Geometry check sheet. Reference: the model listing, model coordinates, mm. Face numbers are marked on the shaded views. A direction names the side the tool comes from. Round coordinates to 2 decimals unless told otherwise and drop trailing zeros. Write each loop counter-clockwise with the first axis right and the second up, starting at its lowest first coordinate (ties: lowest second). Pieces come first, ordered by that corner, then holes. Notation, with made-up numbers: (64, -2) -> (120, -2) arc R19 ccw to (120, 33) -> close; hole circle Ø1 at (-35.5, 8.5). An arc over 180 degrees is marked (long way). One line per question, with ' | ' between items.
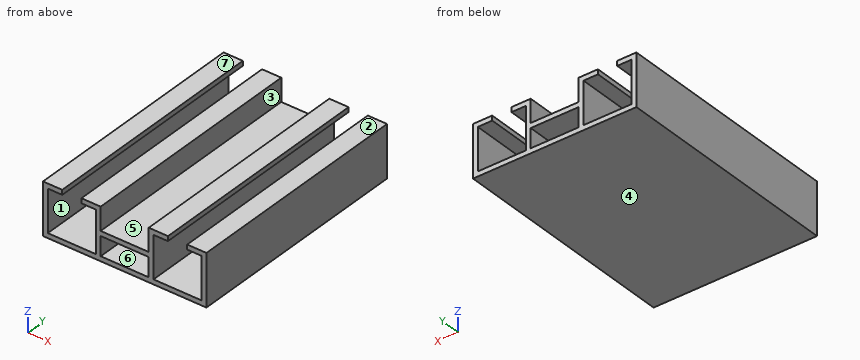
```python
from build123d import *

# Parameters (mm, degrees)
F0_W     = 25
F0_H     = 10
F1_DEPTH = 60


with BuildPart() as f1:
    # F0 (on Front) → F1 (new body, symmetric)
    with BuildSketch(Plane.XZ):
        Polygon((42.5, -17.5), (42.5, 9.5), (32.5, 9.5), (32.5, 7), (40, 7), (40, -15), (15, -15), (15, 7), (22.5, 7), (22.5, 9.5), (12.5, 9.5), (12.5, -2.5), (-12.5, -2.5), (-12.5, 9.5), (-22.5, 9.5), (-22.5, 7), (-15, 7), (-15, -15), (-40, -15), (-40, 7), (-32.5, 7), (-32.5, 9.5), (-42.5, 9.5), (-42.5, -17.5), align=None)
        with Locations((0, -10)):
            Rectangle(F0_W, F0_H, mode=Mode.SUBTRACT)
    extrude(amount=F1_DEPTH, both=True)


solid = f1.part
```
(1) Sectioned sample at A-A on z = -7.75. Record the cut outline in (x, y), then the cut area to 3 significant figures.
Resolved:
outline: (-42.5, -60) -> (-40, -60) -> (-40, 60) -> (-42.5, 60) -> close; (-15, -60) -> (-12.5, -60) -> (-12.5, 60) -> (-15, 60) -> close; (12.5, -60) -> (15, -60) -> (15, 60) -> (12.5, 60) -> close; (40, -60) -> (42.5, -60) -> (42.5, 60) -> (40, 60) -> close | area: 1,200 mm2
(2) Material ranges on line 1 (X direction, y = 48, z = 8.75); line 2 (X direction, y = 38.5, z = -11.25); line 3 (X direction, y = 17, z = -4.5), recorded low to high.
Resolved:
line 1: x = -42.5 to -32.5, -22.5 to -12.5, 12.5 to 22.5, 32.5 to 42.5 | line 2: x = -42.5 to -40, -15 to -12.5, 12.5 to 15, 40 to 42.5 | line 3: x = -42.5 to -40, -15 to 15, 40 to 42.5
(3) Access from +Z, -Z, +X, -X, +Y, -Y to the whole of each face (thin tool, end or side, straight path). Record for the marked faces 5, 6 and 7.
Resolved:
face 5: +Z, +Y, -Y | face 6: +Y, -Y | face 7: +Z, +X, -X, +Y, -Y
(4) Draft check along Z on the marked faces 1, 2, 3 and 4. Enter one of: +Z half, -Z half, draft (parallel to the pull), parting line (faces both ways), or undercut.
Resolved:
face 1: undercut | face 2: +Z half | face 3: draft | face 4: -Z half
(5) Sectioned sample at C-C on y = -7.5. Record the cut outline in (x, z), then the cut area to 3 significant figures.
Resolved:
outline: (-42.5, -17.5) -> (42.5, -17.5) -> (42.5, 9.5) -> (32.5, 9.5) -> (32.5, 7) -> (40, 7) -> (40, -15) -> (15, -15) -> (15, 7) -> (22.5, 7) -> (22.5, 9.5) -> (12.5, 9.5) -> (12.5, -2.5) -> (-12.5, -2.5) -> (-12.5, 9.5) -> (-22.5, 9.5) -> (-22.5, 7) -> (-15, 7) -> (-15, -15) -> (-40, -15) -> (-40, 7) -> (-32.5, 7) -> (-32.5, 9.5) -> (-42.5, 9.5) -> close; hole (-12.5, -15) -> (12.5, -15) -> (12.5, -5) -> (-12.5, -5) -> close | area: 595 mm2
(6) Go/stop test with a flat-tipped pin: pin 1 (7.5 mm diameter, centred on x = -3, y = -5, fed in from +Z). Record where the tip stops, or that it passes through.
Resolved:
pin 1: stops at z = -2.5
(7) Sectioned sample at B-B on x = -5.5. Record the cut outline in (y, z), then the cut area to 3 significant figures.
Resolved:
outline: (-60, -17.5) -> (60, -17.5) -> (60, -15) -> (-60, -15) -> close; (-60, -5) -> (60, -5) -> (60, -2.5) -> (-60, -2.5) -> close | area: 600 mm2
